Drawing for the job (mm, zero at the part's lowest x, y, z). Give positions to 0.01 mm unless a question says otherwise; leave off trailing zeros. Order: outer loops, then holes, each group sorted by start corner. A loop starts at its lowest first (then second) coordinate and runs counter-clockwise, first axis right, second up. Notation, with made-up numbers: (78, 46) - (131, 46) arc R31 ccw to (131, 74) - close; hole circle Ø3 at (44.25, 21). An arc over 180 degrees is marked (long way). Use CSV: the item, a comma, the result in double quotes. Start each with the question number.
(1) Band-saw the part on A-A, the plane y = 48.8. Give the cut face in (x, z).
(2) Probe L1, parallel to Y at x = 2.5, z = 4.25; L2, parallel to Z at x = 4.75, y = 12.8; L3, parallel to Z at x = 1.5, y = 47. List the from-to ranges inside material, lowest first.
(3) Drop a flat-ended pin along its axis: pin 1 Ø4 at (x, z) = (2.5, 3) entering from -Y. Give the stop position or say it passes through.
(4) Band-saw the part on B-B, the plane x = 6.75. Give the cut face in (y, z).
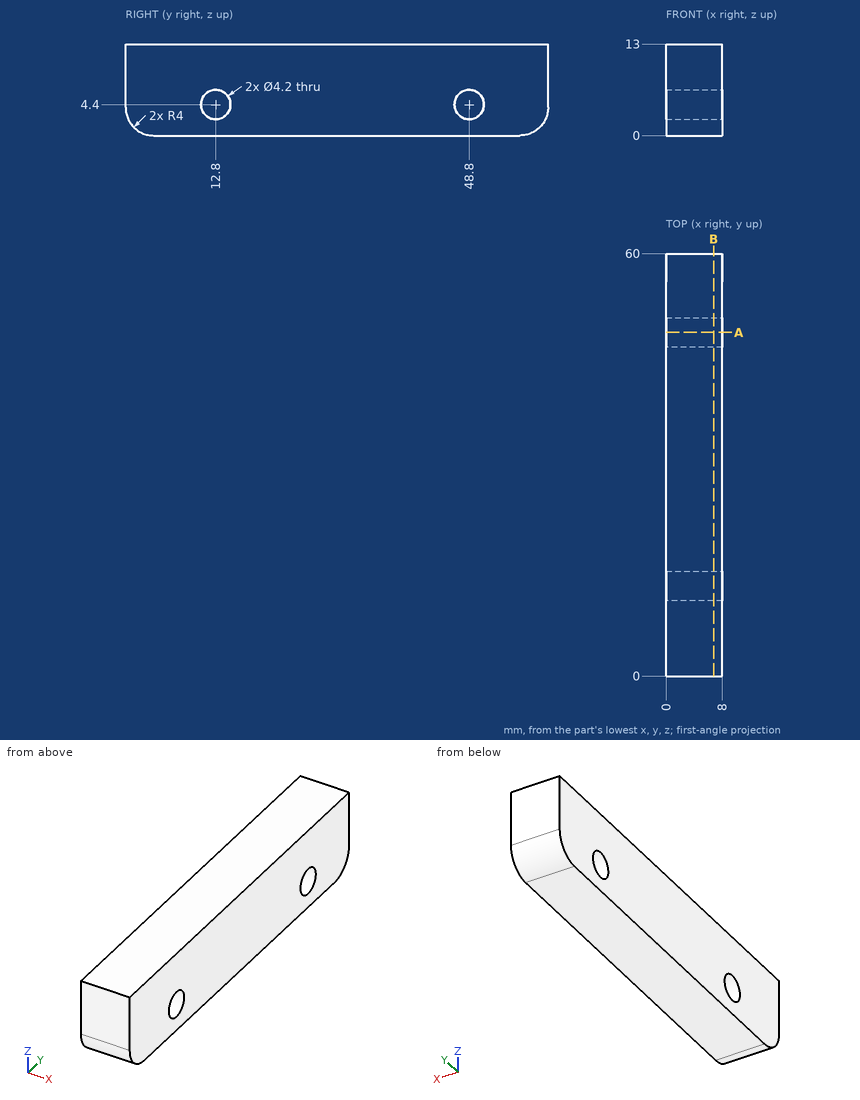
Answer block:
1,outline,"(0, 0) - (8, 0) - (8, 2.3) - (0, 2.3) - close; (0, 6.5) - (8, 6.5) - (8, 13) - (0, 13) - close"
2,L1,"y = 0 to 10.71, 14.89 to 46.71, 50.89 to 60"
2,L2,"z = 0 to 2.3, 6.5 to 13"
2,L3,"z = 0 to 3.32, 5.48 to 13"
3,pin 1,"stops at y = 0"
4,outline,"(0, 4) arc R4 ccw to (4, 0) - (56, 0) arc R4 ccw to (60, 4) - (60, 13) - (0, 13) - close; hole circle Ø4.2 at (12.8, 4.4); hole circle Ø4.2 at (48.8, 4.4)"
